Job drawing, mm, ordinate dimensions from the low corner. One solid piece. A direction names the side the tool comes from. Coordinates: 2 decimals unless noted, no trailing zeros. Order: outer loops, then holes, each group sorted by start corner. A loop starts at its lowest first (then second) coordinate and runs counter-clockwise, first axis right, second up. Notation, with made-up numbers: (39.25, 70.5) -> (58.25, 70.5) arc R17 ccw to (58.25, 95.5) -> close; hole circle Ø6 at (-28.5, 31). An arc over 180 degrees is marked (long way). Use CSV: the item, a comma, the result in double quotes. Start each with the question number.
(1) Cut at C-C on z = 94. Write the cut outline in (x, y), plus the area to 3 significant figures.
(2) Cut at A-A on x = 27. Write the cut outline in (y, z).
(3) Pull direction X, two halves, no side cores. Call the marked faces 3, 4 and 5: pulls with the +X half, pulls with the -X half, needs draft (parallel to the pull), parting line crosses it, or undercut.
(4) Cut at B-B on y = 49.5. Write the cut outline in (x, z), plus the area to 3 significant figures.
(5) Tool access for the marked faces 1 and 2: list every direction of +Z, -Z, +X, -X, +Y, -Y with a clear straight run to the whole face (end or side of a thin tool).
(6) Pin check, flat tip, straight feed: pin 1 Ø1 at (y, z) = (8.5, 35.5) entering from +X. Stop position of the tip, or through.
(7) Probe L1, parallel to X at y = 50.5, z = 80; L2, parallel to Y at x = 48, z = 53; L3, parallel to X at y = 64, z = 37. List the from-to ranges inside material, lowest first.
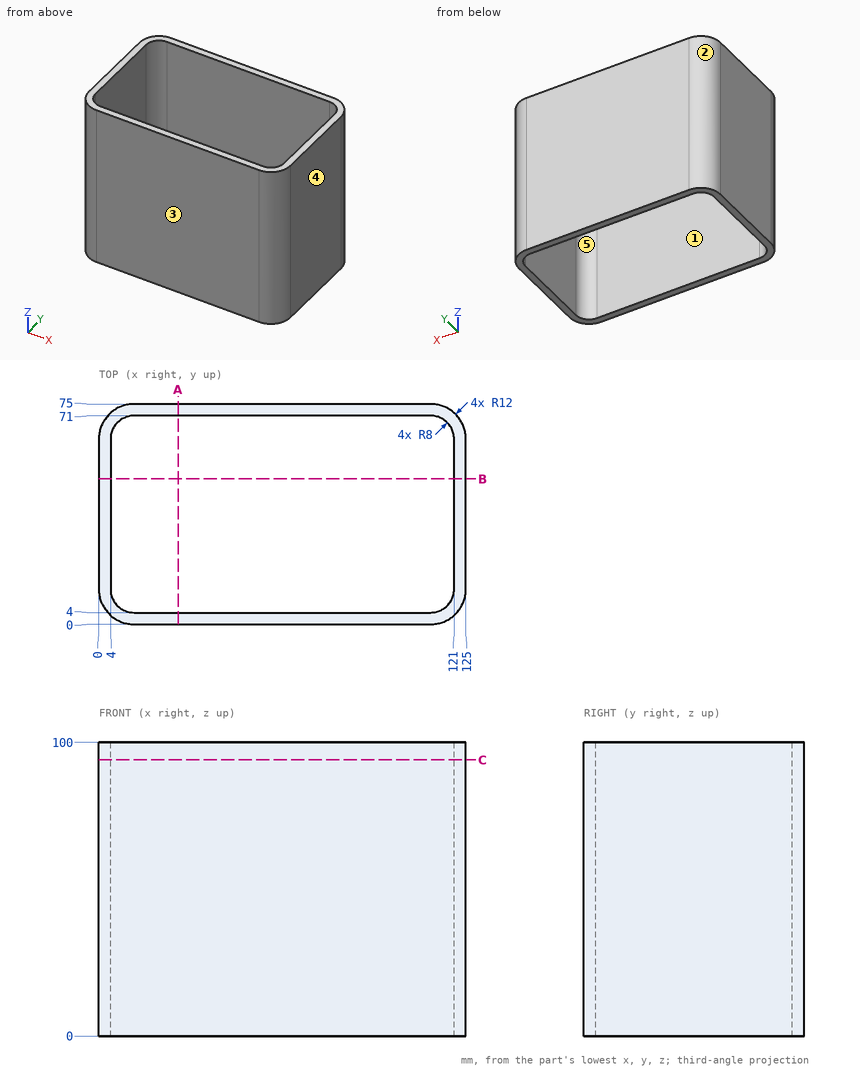
Outcome:
1,outline,"(0, 12) arc R12 ccw to (12, 0) -> (113, 0) arc R12 ccw to (125, 12) -> (125, 63) arc R12 ccw to (113, 75) -> (12, 75) arc R12 ccw to (0, 63) -> close; hole (4, 12) arc R8 ccw to (12, 4) -> (113, 4) arc R8 ccw to (121, 12) -> (121, 63) arc R8 ccw to (113, 71) -> (12, 71) arc R8 ccw to (4, 63) -> close"
1,area,"1,470 mm2"
2,outline,"(0, 0) -> (4, 0) -> (4, 100) -> (0, 100) -> close; (71, 0) -> (75, 0) -> (75, 100) -> (71, 100) -> close"
3,face 3,"needs draft"
3,face 4,"pulls with the +X half"
3,face 5,"undercut"
4,outline,"(0, 0) -> (4, 0) -> (4, 100) -> (0, 100) -> close; (121, 0) -> (125, 0) -> (125, 100) -> (121, 100) -> close"
4,area,"800 mm2"
5,face 1,"+Z, -Z"
5,face 2,"+Z, -Z, -X, +Y"
6,pin 1,"x = 124.62"
7,L1,"0 to 4, 121 to 125"
7,L2,"0 to 4, 71 to 75"
7,L3,"0.04 to 4.06, 120.94 to 124.96"
